Verification items for this drawing (mm, ordinates from the low corner). A direction names the side the tool comes from. Round coordinates to 2 decimals unless told otherwise and drop trailing zeros. Order: outer loops, then holes, each group sorted by start corner. A loop starts at its lowest first (then second) coordinate and runs counter-clockwise, first axis right, second up. Notation, with made-up numbers: (-14.75, 64) - (15.25, 64) arc R12 ccw to (15.25, 68) - close; hole circle Ø5 at (-23.5, 12). An arc over 180 degrees is marked (long way). One line per question, with ' | ' between items. Start each with the question number.
Q1. Mould release check, pull along X, two halves, no side actions. Record for the marked faces 1, 2, 3 and 4: +X half, -X half, draft (parallel to the pull), parting line (faces both ways), or undercut.
Q2. Sectioned sample at C-C, the plane x = 19. Enter the section's corners in (y, z).
Q3. Tool access check on the marked faces 5 and 6. Record the directions out of +Z, -Z, +X, -X, +Y, -Y that give a thin tool (end or side, any length) a straight path to the whole face; none if there is none.
Q4. Sectioned sample at D-D, the plane z = 22. Enter the section's corners in (x, y), then the cut area to 3 significant figures.
Q5. Material ranges on line 1 along Z through (x, y) = (11.5, 39.65); line 2 along Z through (x, y) = (11.5, 37.8); line 3 along X through (y, z) = (39, 3), recorded low to high.
Q6. Gauge pin test, flat ends, axial feed: P1, Ø1.5, axis at x = 22.5, y = 34, coming from the +Z side; P2, Ø9, axis at x = 43, z = 35, coming from the +Y side; P3, Ø4, axis at y = 11, z = 37, coming from the +X side; P4, Ø4.5, axis at x = 11.5, z = 5.5, coming from the -Y side. Record the tip position at first contact, or that the pin passes through.
Q7. Sectioned sample at A-A, the plane x = 42.5. Enter the section's corners in (y, z), then the cut area to 3 significant figures.
Q8. Sectioned sample at B-B, the plane z = 5.5. Enter the section's corners in (x, y).
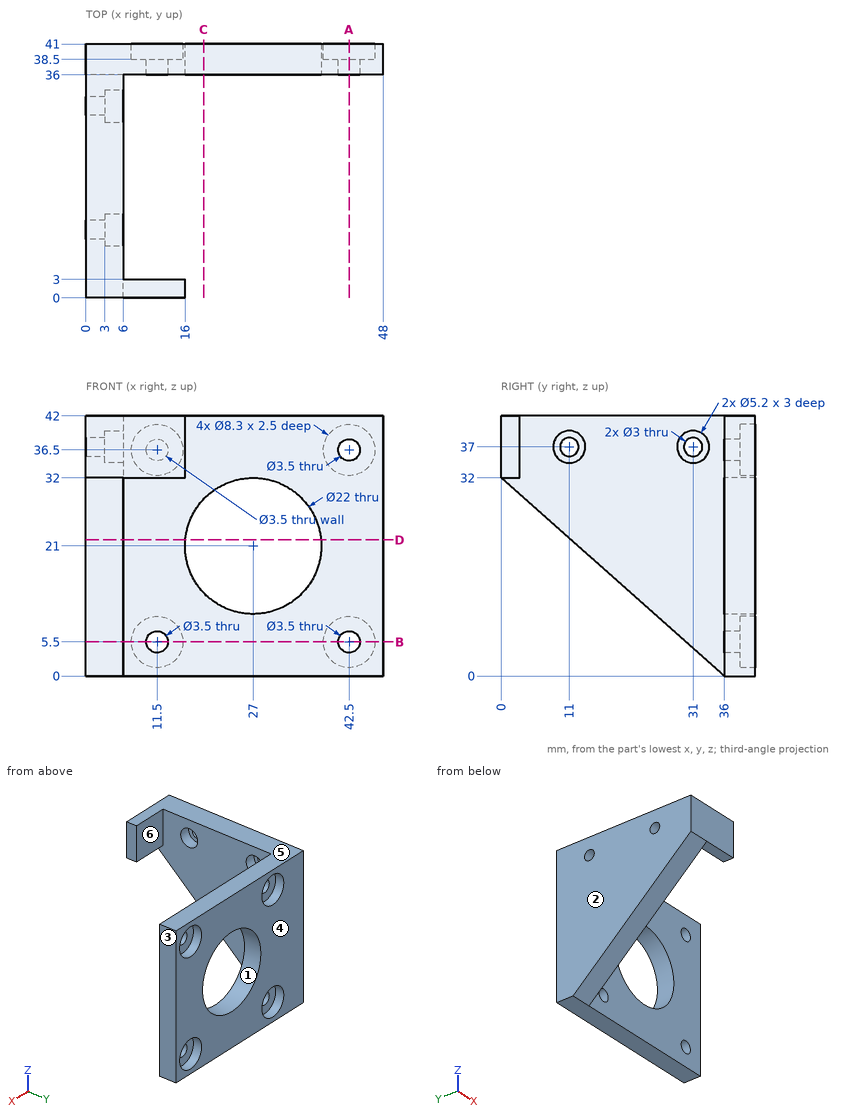
Determined:
1) face 1: undercut | face 2: -X half | face 3: +X half | face 4: draft
2) outline: (36, 0) - (41, 0) - (41, 13.45) - (36, 13.45) - close; (36, 28.55) - (41, 28.55) - (41, 42) - (36, 42) - close
3) face 5: +Z, +X, -X, +Y, -Y | face 6: +Z, -Z, +X
4) outline: (0, 11.25) - (6, 11.25) - (6, 36) - (16.05, 36) - (16.05, 41) - (0, 41) - close; (37.95, 36) - (48, 36) - (48, 41) - (37.95, 41) - close | area: 279 mm2
5) line 1: z = 0 to 1.35, 9.65 to 32.35, 40.65 to 42 | line 2: z = 0 to 3.75, 7.25 to 34.75, 38.25 to 42 | line 3: x = 0 to 8.19, 14.81 to 39.19, 45.81 to 48
6) P1: passes through | P2: stops at y = 41 | P3: stops at x = 3 | P4: stops at y = 36
7) outline: (36, 0) - (41, 0) - (41, 1.35) - (38.5, 1.35) - (38.5, 3.75) - (36, 3.75) - close; (36, 7.25) - (38.5, 7.25) - (38.5, 9.65) - (41, 9.65) - (41, 32.35) - (38.5, 32.35) - (38.5, 34.75) - (36, 34.75) - close; (36, 38.25) - (38.5, 38.25) - (38.5, 40.65) - (41, 40.65) - (41, 42) - (36, 42) - close | area: 151 mm2
8) outline: (0, 29.81) - (6, 29.81) - (6, 36) - (9.75, 36) - (9.75, 38.5) - (7.35, 38.5) - (7.35, 41) - (0, 41) - close; (13.25, 36) - (40.75, 36) - (40.75, 38.5) - (38.35, 38.5) - (38.35, 41) - (15.65, 41) - (15.65, 38.5) - (13.25, 38.5) - close; (44.25, 36) - (48, 36) - (48, 41) - (46.65, 41) - (46.65, 38.5) - (44.25, 38.5) - close
